CAD build for the part. Positions are in the model's coordinates, mm. Face numbers are marked on the shaded views. Round coordinates to 2 decimals unless told otherwise and drop trailing zeros. Order: outer loops, then holes, each group sorted by start corner. A loop starts at its lowest first (then second) coordinate and runs counter-clockwise, first axis right, second up. Notation, with made-up numbers: (-2.75, 76) -> (29.25, 76) arc R6 cw to (29.25, 81) -> close; hole circle Ø2 at (-1.75, 19). An arc over 180 degrees is marked (long way). Return JSON: item names as keys, results as strings. Group by question number.
Q1. Probe line 1 along X through (y, z) = (-29.5, 17.75); line 2 along X through (y, z) = (22.5, 4.75); line 3 along Y through (x, z) = (33.5, 16.5). List the from-to ranges inside material, lowest first.
Q2. Mould opens along Y. For the marked faces 1, 2 and 3 say: +Y half, -Y half, draft (parallel to the pull), parting line (faces both ways), or undercut.
Q3. Cut at A-A (x = 0). Write the cut outline in (y, z) (3 decimals), then the cut area to 3 significant figures.
Q4. Flat gauge pins, fed straight in: pin 1 (10 mm diameter, centred on x = -15, z = 16.5, fed in from -Y); pin 2 (4 mm diameter, centred on y = 14.5, z = 13.5, fed in from -X); pin 3 (1 mm diameter, centred on y = -18.5, z = 18.5, fed in from +X); pin 4 (3 mm diameter, centred on x = -29.7, y = -29.7, fed in from -Z). Where does each tip first touch, or does it go through?
Q5. Cut at D-D (z = 4.75). Count the separate pieces of the cut face and the enclosed holes in it, then the cut area to 3 significant figures.
Q6. Cut at B-B (x = 25). Write the cut outline in (y, z), then the cut area to 3 significant figures.
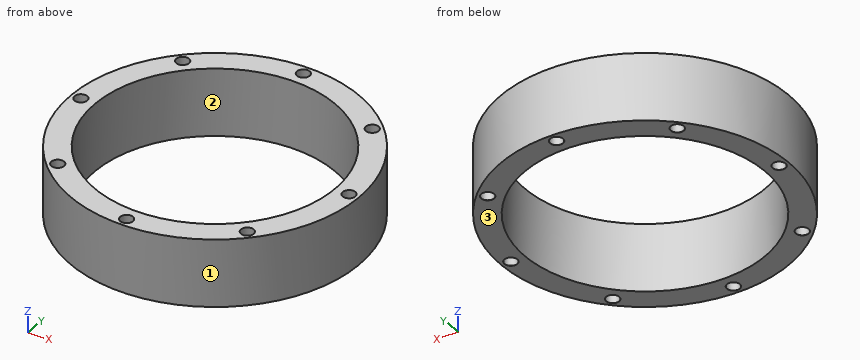
from build123d import *

# Parameters (mm, degrees)
SKETCH1_R                       = 45
SKETCH1_R_2                     = 37.5
BOSS_EXTRUDE1_DEPTH             = 21
F_4_0MM_DOWEL_HOLE1_D           = 4
F_4_0MM_DOWEL_HOLE1_CSINK_D     = 4.05
F_4_0MM_DOWEL_HOLE1_CSINK_ANGLE = 90


with BuildPart() as part:
    # Sketch1 → Boss-Extrude1 (new body)
    with BuildSketch(Plane.XY):
        with Locations(Location((0, 0, 0), (0, 0, 180))):
            Circle(SKETCH1_R)
        with Locations(Location((0, 0, 0), (0, 0, 180))):
            Circle(SKETCH1_R_2, mode=Mode.SUBTRACT)
    extrude(amount=BOSS_EXTRUDE1_DEPTH)

    # Ø4.0mm Dowel Hole1 (through all)
    with Locations(Plane(origin=(0, 0, 0), x_dir=(-1, 0, 0), z_dir=(0, 0, -1))):
        with Locations((29.69848481, 29.69848481), (0, 42), (-29.69848481, 29.69848481), (-42, 0), (-29.69848481, -29.69848481), (0, -42), (29.69848481, -29.69848481), (42, 0)):
            CounterSinkHole(F_4_0MM_DOWEL_HOLE1_D / 2, F_4_0MM_DOWEL_HOLE1_CSINK_D / 2, counter_sink_angle=F_4_0MM_DOWEL_HOLE1_CSINK_ANGLE)


solid = part.part
Solution:
{
 "1": {"line 1": "x = -33.98 to -31.69, -27.71 to -23.15, 23.15 to 27.71, 31.69 to 33.98", "line 2": "x = -38.97 to -30, 30 to 38.97", "line 3": "y = -30.05 to -16.85, 16.85 to 30.05"},
 "2": {"face 1": "parting line", "face 2": "undercut", "face 3": "draft"},
 "3": {"outline": "(-45, 0) -> (-44.025, 0) -> (-44, 0.025) -> (-44, 21) -> (-45, 21) -> close; (-40, 0.025) -> (-39.975, 0) -> (-37.5, 0) -> (-37.5, 21) -> (-40, 21) -> close; (37.5, 0) -> (39.975, 0) -> (40, 0.025) -> (40, 21) -> (37.5, 21) -> close; (44, 0.025) -> (44.025, 0) -> (45, 0) -> (45, 21) -> (44, 21) -> close", "area": "147 mm²"},
 "4": {"pin 1": "stops at y = -43.87", "pin 2": "stops at x = -43.23", "pin 3": "stops at x = 41.24", "pin 4": "passes through"},
 "5": {"separate pieces": "1", "enclosed holes": "9", "area": "1,840 mm²"},
 "6": {"outline": "(-37.42, 0) -> (-27.95, 0) -> (-27.95, 21) -> (-37.42, 21) -> close; (27.95, 0) -> (37.42, 0) -> (37.42, 21) -> (27.95, 21) -> close", "area": "398 mm²"}
}
